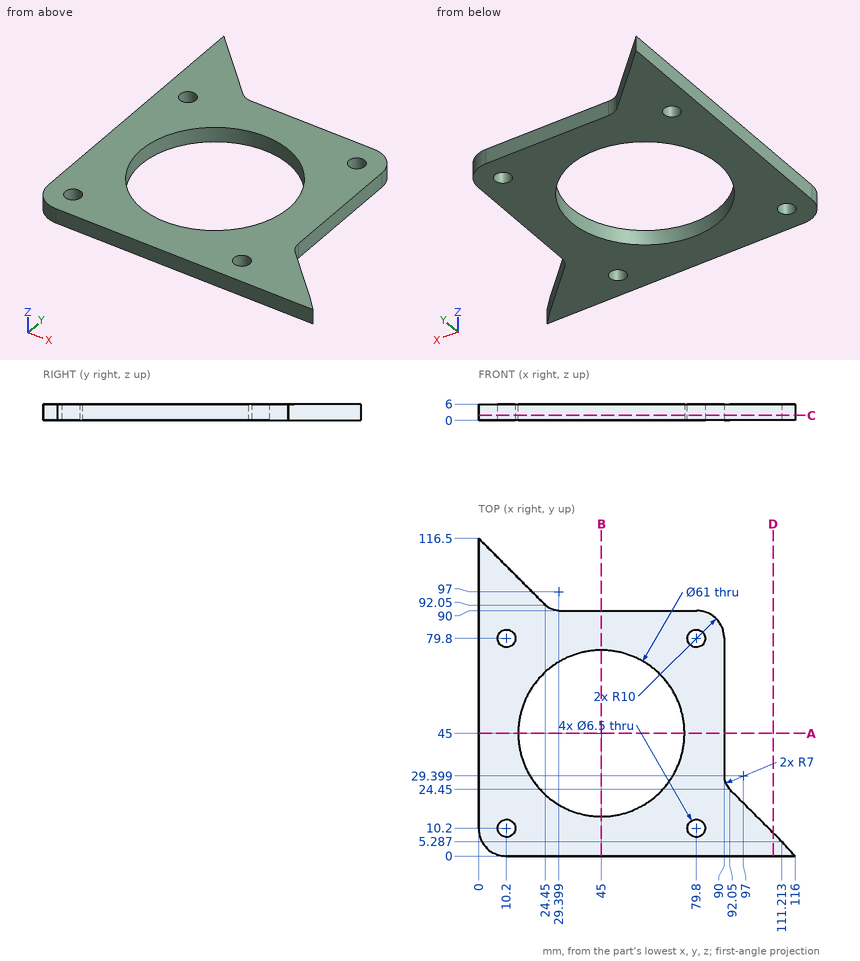
Geometry: see drawing. Coordinates: mm, zero at the bounding-box minimum. Give positions to 0.01 mm unless a question says otherwise; leave off trailing zeros. Write each loop counter-clockwise with the first axis right and the second up, starting at its lowest first coordinate (ties: lowest second). Pieces come first, ordered by that corner, then holes. Notation, with made-up numbers: (69.25, 34.5) - (86.25, 34.5) arc R15 ccw to (86.25, 43.5) - close; hole circle Ø1 at (38.5, 51.25). An arc over 180 degrees is marked (long way). Return JSON: item names as keys, results as strings. Group by question number.
1) Section D-D on x = 108. Return the cut outline in (y, z).
2) Section A-A on y = 45. Return the cut outline in (x, z).
3) First-contact query: P1, Ø3, axis at y = 52.5, z = 4, coming from the +X side; P2, Ø3, axis at x = 87.5, z = 5, coming from the +Y side. Flat tips, straight axial feed; report the tip coordinate or a pass-through.
4) Line query: line 1 (Y direction, x = 79.8, z = 1.55); line 2 (Y direction, x = 45, z = 1.3); line 3 (Y direction, x = 10.2, z = 1.8). Output: solid intervals per line, ascending.
5) Section C-C on z = 1.85. Return the cut outline in (x, y).
Filled in:
{
 "1": {"outline": "(0, 0) - (8.5, 0) - (8.5, 6) - (0, 6) - close"},
 "2": {"outline": "(0, 0) - (14.5, 0) - (14.5, 6) - (0, 6) - close; (75.5, 0) - (90, 0) - (90, 6) - (75.5, 6) - close"},
 "3": {"P1": "stops at x = 90", "P2": "stops at y = 88"},
 "4": {"line 1": "y = 0 to 6.95, 13.45 to 76.55, 83.05 to 90", "line 2": "y = 0 to 14.5, 75.5 to 90", "line 3": "y = 0 to 6.95, 13.45 to 76.55, 83.05 to 106.3"},
 "5": {"outline": "(0, 10) arc R10 ccw to (10, 0) - (116, 0) - (111.21, 5.29) - (92.05, 24.45) arc R7 cw to (90, 29.4) - (90, 80) arc R10 ccw to (80, 90) - (29.4, 90) arc R7 cw to (24.45, 92.05) - (0, 116.5) - close; hole circle Ø6.5 at (10.2, 10.2); hole circle Ø6.5 at (10.2, 79.8); hole circle Ø61 at (45, 45); hole circle Ø6.5 at (79.8, 10.2); hole circle Ø6.5 at (79.8, 79.8)"}
}
